Check sheet for the drawn part. Datum: minimum x, y, z corner. Units: mm. Coordinates: 2 decimals unless noted, no trailing zeros. Loops run counter-clockwise (first coordinate to the right, second up) from the corner with the lowest first, then second, coordinate; pieces in that order, holes last.
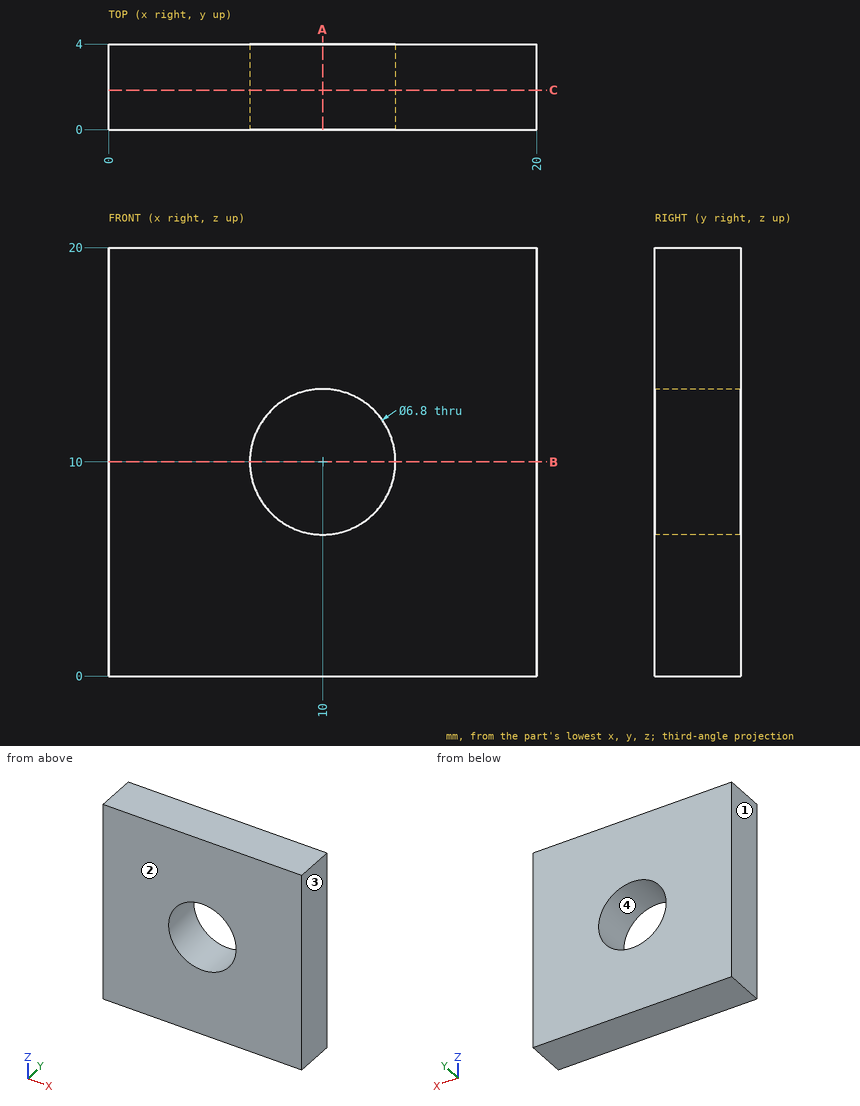
1) Section check B-B on z = 10. Enter the section's corners in (x, y), plus the area to 3 significant figures.
Answer sheet:
outline: (0, 0) - (6.6, 0) - (6.6, 4) - (0, 4) - close; (13.4, 0) - (20, 0) - (20, 4) - (13.4, 4) - close
area: 52.8 mm2
2) Section check C-C on y = 1.85. Enter the section's corners in (x, z).
Answer sheet:
outline: (0, 0) - (20, 0) - (20, 20) - (0, 20) - close; hole circle Ø6.8 at (10, 10)
3) Scan lines: line 1 (Z direction, x = 10, y = 2.3); line 2 (Z direction, x = 12, y = 2.8). Record each from-to range of solid material in increasing order.
Answer sheet:
line 1: z = 0 to 6.6, 13.4 to 20
line 2: z = 0 to 7.25, 12.75 to 20
4) Mould release check, pull along X, two halves, no side actions. Record for the marked faces 1, 2, 3 and 4: +X half, -X half, draft (parallel to the pull), parting line (faces both ways), or undercut.
Answer sheet:
face 1: -X half
face 2: draft
face 3: +X half
face 4: undercut
5) Depth check by flat-ended pin: pin 1 (1.5 mm diameter, centred on y = 1, z = 6.5, fed in from -X). Enter the tip coordinate at first touch or a pass-through.
Answer sheet:
pin 1: stops at x = 0
6) Section check A-A on x = 10. Enter the section's corners in (y, z), plus the area to 3 significant figures.
Answer sheet:
outline: (0, 0) - (4, 0) - (4, 6.6) - (0, 6.6) - close; (0, 13.4) - (4, 13.4) - (4, 20) - (0, 20) - close
area: 52.8 mm2
